```python
from build123d import *

# Parameters (mm, degrees)
SKETCH_1_W          = 18
SKETCH_1_H          = 2
SKETCH_1_W_2        = 2
SKETCH_1_H_2        = 20
EXTRUDE_1_DEPTH     = 55
SKETCH_2_R          = 1.566180025
CUT_EXTRUDE_1_DEPTH = 10


with BuildPart() as part:
    # Эскиз1 → Бобышка-Вытянуть1 (new body)
    with BuildSketch(Plane.XY):
        with Locations((-9, 1)):
            Rectangle(SKETCH_1_W, SKETCH_1_H)
        with Locations((1, 10)):
            Rectangle(SKETCH_1_W_2, SKETCH_1_H_2)
    extrude(amount=EXTRUDE_1_DEPTH)

    # Эскиз2 → Вырез-Вытянуть1 (cut)
    with BuildSketch(Plane.XZ):
        with Locations((-10.550157234, 7)):
            Circle(SKETCH_2_R)
        with Locations((-10.550157234, 48)):
            Circle(SKETCH_2_R)
    extrude(amount=-CUT_EXTRUDE_1_DEPTH, mode=Mode.SUBTRACT)


solid = part.part
```
Input: part model. Units: mm. Frame: model coordinates. A direction names the side the tool comes from. Give positions to 0.01 mm unless a question says otherwise; leave off trailing zeros. Order: outer loops, then holes, each group sorted by start corner. A loop starts at its lowest first (then second) coordinate and runs counter-clockwise, first axis right, second up.
1. Mould query, pull axis X, two halves, no side actions, for faces 3 (the flat face through (-4, 1, 0)), 4 (the cylindrical face through (-10.89, 0.99, 5.47)), 5 (the flat face through (0, 11, 27)). Classes: released by +X, released by -X, zero draft, split by the parting line, or undercut.
Derived:
face 3: zero draft
face 4: undercut
face 5: released by -X
2. Section A-A on z = 7. Return the cut outline in (x, y), and give its area (3 significant figures).
Derived:
outline: (-18, 0) - (-12.12, 0) - (-12.12, 2) - (-18, 2) - close; (-8.98, 0) - (2, 0) - (2, 20) - (0, 20) - (0, 2) - (-8.98, 2) - close
area: 69.7 mm2
3. Section B-B on x = -9.75. Return the cut outline in (y, z).
Derived:
outline: (0, 0) - (2, 0) - (2, 5.65) - (0, 5.65) - close; (0, 8.35) - (2, 8.35) - (2, 46.65) - (0, 46.65) - close; (0, 49.35) - (2, 49.35) - (2, 55) - (0, 55) - close
4. Section D-D on y = 12. Return the cut outline in (x, z).
Derived:
outline: (0, 0) - (2, 0) - (2, 55) - (0, 55) - close
5. Pin query (flat end, axial travel): pin 1 (2 mm diameter, centred on y = 4.5, z = 31, fed in from -X); pin 2 (3.5 mm diameter, centred on x = -10.55, z = 48, fed in from +Y). Return the tip coordinate at first contact, or that it passes through.
Derived:
pin 1: stops at x = 0
pin 2: stops at y = 2
6. Section C-C on z = 29. Return the cut outline in (x, y), and give its area (3 significant figures).
Derived:
outline: (-18, 0) - (2, 0) - (2, 20) - (0, 20) - (0, 2) - (-18, 2) - close
area: 76.0 mm2
7. Material intervals for L1, parallel to Y at x = -4.25, z = 22.5, sorted ascending.
Derived:
L1: y = 0 to 2
8. Reachability of faces 1 (the flat face through (-9, 2, 27)), 2 (the cylindrical face through (-10.754, 0.986, 49.553)) from +Z, -Z, +X, -X, +Y, -Y: full face, straight path, thin tool, end or side. Return the list, or none.
Derived:
face 1: +Z, -Z, -X, +Y
face 2: +Y, -Y
